Autodesk Inventor part; units mm, degrees
ref_plane "YZ Plane" through (0, 0, 0) normal (1, 0, 0) x (0, 1, 0)
ref_plane "XZ Plane" through (0, 0, 0) normal (0, 1, 0) x (-1, 0, 0)
ref_plane "XY Plane" through (0, 0, 0) normal (0, 0, 1) x (1, 0, 0)
sketch "Sketch1" plane through (0, 0, 0) normal (0, 1, 0) x (-1, 0, 0)
  line L0 (0, 0) -> (55, 0)
  line L1 (55, 0) -> (55, -63)
  line L2 (55, -63) -> (0, -63)
  line L3 (0, -63) -> (0, 0)
  dimension "d0" = 55
  dimension "d1" = 63
extrude "Extrusion1" add sketch "Sketch1" along normal blind 3
sketch "Sketch2" plane through (0, 0, 0) normal (0, -1, 0) x (1, 0, 0)
  line L0 (0, 0) -> (-10, 0)
  line L1 (-10, 0) -> (-10, -3)
  line L2 (-10, -3) -> (0, -3)
  line L3 (0, -3) -> (0, 0)
  line L4 (-55, -63) -> (-55, 0)
  line L5 (-55, 0) -> (-45, 0)
  line L6 (-45, 0) -> (-45, -3)
  line L7 (-45, -3) -> (-55, -3)
  line L8 (-55, -3) -> (-55, 0)
  line L9 (-55, -63) -> (-45, -63)
  line L10 (-45, -63) -> (-45, -60)
  line L11 (-45, -60) -> (-55, -60)
  line L12 (-55, -60) -> (-55, -63)
  line L13 (0, -63) -> (-10, -63)
  line L14 (-10, -63) -> (-10, -60)
  line L15 (-10, -60) -> (0, -60)
  line L16 (0, -60) -> (0, -63)
  dimension "d4" = 10
  dimension "d5" = 3
  dimension "d6" = 10
  dimension "d7" = 3
  dimension "d8" = 10
  dimension "d9" = 3
  dimension "d10" = 10
  dimension "d11" = 3
extrude "Extrusion2" add sketch "Sketch2" along normal blind 7
sketch "Sketch3" plane through (-55, 3, 0) normal (0, 0, 1) x (1, 0, 0)
  line L0 (10, -10) -> (0, -10)
  line L1 (0, -10) -> (5, -10)
  line L2 (5, -10) -> (5, -6)
  line L3 (5, -6) -> (0, -6)
  line L4 (0, -6) -> (0, -10)
  line L5 (45, -3) -> (45, -10)
  line L6 (45, -10) -> (50, -10)
  line L7 (50, -10) -> (50, -6)
  line L8 (50, -6) -> (45, -6)
  line L9 (45, -6) -> (45, -10)
  circle A0 centre (5, -6) radius 2
  circle A1 centre (50, -6) radius 2
  point P0 (55, -3)
  dimension "d14" = 5
  dimension "d15" = 4
  dimension "d16" = 5
  dimension "d17" = 4
  dimension "d18" = 4
  dimension "d19" = 4
extrude "Extrusion3" cut sketch "Sketch3" against normal up to surface (63 mm away) contours A0 L3 L2 | L2 L3 A0 | A1 L7 L8 | L8 L7 A1
fillet "Fillet1" radius 4 8 edges at (0, -7, -1.5) (-10, -7, -61.5) (0, -7, -61.5) (-45, -7, -61.5) (-55, -7, -61.5) (-45, -7, -1.5) (-55, -7, -1.5) (-10, -7, -1.5)
sketch "Sketch4" plane through (0, 3, 0) normal (0, 1, 0) x (1, 0, 0)
  line L0 (0, 0) -> (15, 0)
  line L1 (15, 0) -> (15, 63)
  line L2 (15, 63) -> (0, 63)
  line L3 (0, 63) -> (0, 0)
  dimension "d23" = 15
  dimension "d24" = 63
extrude "Extrusion4" add sketch "Sketch4" against normal blind 3
sketch "Sketch5" plane through (0, 3, 0) normal (0, 1, 0) x (1, 0, 0)
  line L0 (14.6866, 62.7723) -> (4.6866, 62.7723)
  line L1 (4.6866, 62.7723) -> (4.6866, 52.7723)
  line L2 (4.6866, 52.7723) -> (14.6866, 52.7723)
  line L3 (14.6866, 52.7723) -> (14.6866, 62.7723)
  line L4 (4.6866, 52.7723) -> (-25.6434, 52.7723)
  line L5 (-25.6434, 52.7723) -> (-25.6434, 37.0423)
  line L6 (-25.6434, 37.0423) -> (4.6866, 37.0423)
  line L7 (4.6866, 37.0423) -> (4.6866, 52.7723)
  circle A0 centre (-25.6434, 52.7723) radius 1
  circle A1 centre (4.6866, 37.0423) radius 1
  circle A2 centre (4.6866, 37.0423) radius 2
  circle A3 centre (-25.6434, 52.7723) radius 2
  point P0 (0, 0)
  dimension "d27" = 10
  dimension "d28" = 10
  dimension "d29" = 30.33
  dimension "d30" = 15.73
  dimension "d31" = 2
  dimension "d32" = 2
  dimension "d33" = 4
  dimension "d34" = 4
extrude "Extrusion5" cut sketch "Sketch5" against normal blind 3 contours A0 L5 L4 | L4 L5 A0 | A1 L6 L7 | L7 L6 A1
sketch "Sketch6" plane through (0, 3, 0) normal (0, 1, 0) x (1, 0, 0)
  line L0 (15, 63) -> (-55, 63)
  line L1 (-55, 63) -> (-55, 53)
  line L2 (-55, 53) -> (-35, 53)
  line L3 (-35, 53) -> (-35, 33)
  line L4 (-35, 33) -> (-55, 33)
  line L5 (-55, 33) -> (-55, 53)
  point P0 (0, 0)
  dimension "d37" = 10
  dimension "d38" = 20
  dimension "d39" = 20
extrude "Extrusion6" cut sketch "Sketch6" against normal blind 3
fillet "Fillet2" radius 4 4 edges at (-35, 1.5, -53) (-35, 1.5, -33) (-55, 1.5, -53) (-55, 1.5, -33)
fillet "Fillet3" radius 4 2 edges at (15, 1.5, 0) (15, 1.5, -63)
sketch "Sketch7" plane through (0, 3, 0) normal (0, 1, 0) x (1, 0, 0)
  line L0 (15, 0) -> (5, 0)
  line L1 (5, 0) -> (5, 10)
  line L2 (5, 10) -> (15, 10)
  line L3 (15, 10) -> (15, 0)
  line L4 (5, 10) -> (-50.626, 10)
  line L5 (-50.626, 10) -> (-50.626, 16.3068)
  line L6 (5, 16.3068) -> (5, 10)
  line L7 (5, 10) -> (-50.626, 10)
  line L8 (-50.626, 10) -> (-50.626, 29.05)
  line L9 (-50.626, 29.05) -> (5, 29.05)
  line L10 (5, 29.05) -> (5, 10)
  circle A0 centre (-50.626, 10) radius 1
  circle A1 centre (-50.626, 29.05) radius 1
  circle A2 centre (5, 29.05) radius 1
  circle A3 centre (5, 10) radius 1
  point P0 (0, 0)
  dimension "d44" = 10
  dimension "d45" = 10
  dimension "d48" = 55.626
  dimension "d49" = 19.05
  dimension "d50" = 2
  dimension "d51" = 2
  dimension "d52" = 2
  dimension "d53" = 2
extrude "Extrusion7" cut sketch "Sketch7" against normal blind 3 contours A3 L4 L1 | L1 L2 A3 | L2 L6 A3 | L4 A3 L6 | A0 L5 L4 | L4 L5 A0 | A2 L9 L10 | L10 L9 A2 | A1 L9 L8 | L8 L9 A1
sketch "Sketch8" plane through (0, 3, 0) normal (0, 1, 0) x (1, 0, 0)
  circle A0 centre (-25.6434, 52.7723) radius 1
  line L0 (-25.6434, 52.7723) -> (-21.6434, 52.7723)
  circle A1 centre (4.6866, 37.0423) radius 1
  line L1 (4.6866, 37.0423) -> (0.6866, 37.0423)
  line L2 (-21.6434, 52.7723) -> (0.6866, 52.7723)
  line L3 (0.6866, 52.7723) -> (0.6866, 37.0423)
  line L4 (0.6866, 37.0423) -> (-21.6434, 37.0423)
  line L5 (-21.6434, 37.0423) -> (-21.6434, 52.7723)
  point P0 (0, 0)
  dimension "d56" = 4
  dimension "d57" = 4
extrude "Extrusion8" cut sketch "Sketch8" against normal blind 10 contours L2 L3 L4 L5
sketch "Sketch9" plane through (0, 3, 0) normal (0, 1, 0) x (1, 0, 0)
  line L0 (-28.7673, 5.8913) -> (-14.8119, 5.8913)
  line L1 (-14.8119, 5.8913) -> (-14.8119, -0.376)
  line L2 (-14.8119, -0.376) -> (-28.7673, -0.376)
  line L3 (-28.7673, -0.376) -> (-28.7673, 5.8913)
  point P0 (0, 0)
extrude "Extrusion9" cut sketch "Sketch9" against normal blind 10
fillet "Fillet4" radius 2 2 edges at (-28.7673, 1.5, 0) (-14.8119, 1.5, 0)
sketch "Sketch11" plane through (0, 3, 0) normal (0, 1, 0) x (1, 0, 0)
  line L0 (17.0243, 33.2031) -> (8.6813, 33.2031)
  line L1 (8.6813, 33.2031) -> (8.6813, 57.6685)
  line L2 (8.6813, 57.6685) -> (17.0243, 57.6685)
  line L3 (17.0243, 57.6685) -> (17.0243, 33.2031)
  point P0 (0, 0)
extrude "Extrusion11" cut sketch "Sketch11" against normal blind 10
fillet "Fillet5" radius 2 2 edges at (15, 1.5, -57.6685) (15, 1.5, -33.2031)
properties part number "servo_driver_support"
Could you check a few things on this model? Use its own coordinates, in mm. A direction names the side the tool comes from. Give positions to 0.01 mm unless a question says otherwise; leave off trailing zeros. Order: outer loops, then holes, each group sorted by start corner. A loop starts at its lowest first (then second) coordinate and runs counter-clockwise, first axis right, second up.
Item 1: If we section it at C-C, the plane y = -6: Write out the boundary of the cut face in (x, z).
Item 2: If we section it at D-D, the plane z = -17.5: Write out the boundary of the cut face in (x, y).
Item 3: For faces 4 (the face through (-51, -5, -60)), 5 (the face through (-14.812, 2, -4)), 6 (the face through (-8.797, -5.859, -1.521)), 7 (the face through (5, 2, -11)), 8 (the face through (-4, -1, 0)), which set-ups out of +Z, -Z, +X, -X, +Y, -Y let a thin tool reach every point of the face, with its end or its side?
Item 4: I need wall thicknesses on line 1 (X direction, y = -3, z = -1.9); line 2 (X direction, y = 0.7, z = -29.05); line 3 (Z direction, x = -49, y = -5.75). Which ranges of each line are inside material? Lowest first, please.
Item 5: If we mould it in two halves opening along X, with no side actions, what happens to faces 1 (the face through (-6.6, -4.2, -1.5)), 2 (the face through (-35, 2, -43)), 3 (the face through (14.43, 1.52, -32.6))? For each: pulls with the +X half, pulls with the -X half, needs draft (parallel to the pull), parting line crosses it, or undercut.
Item 6: If we section it at B-B, the plane x = -25.5: Write out the boundary of the cut face in (y, z), plus the area to 3 significant figures.
Item 7: If we section it at A-A, the plane z = -10: Write out the boundary of the cut face in (x, y).
Item 8: I'm going to push flat-ended pins straight in: pin 1 (12 mm diameter, centred on x = -28.5, z = -56, fed in from -Y); pin 2 (1.5 mm diameter, centred on y = 2, z = -39.5, fed in from +X); pin 3 (3.5 mm diameter, centred on y = 1, z = -42, fed in from -X); pin 4 (1.6 mm diameter, centred on x = 4.69, z = -37.04, fed in from -Y). Where does each tip first touch, or does it pass through?
Values:
1. outline: (-53.65, -63) - (-46.35, -63) - (-46.35, -60) - (-53.65, -60) - close; (-53.65, -3) - (-46.35, -3) - (-46.35, 0) - (-53.65, 0) - close; (-8.65, -63) - (-1.35, -63) - (-1.35, -60) - (-8.65, -60) - close; (-8.65, -3) - (-1.35, -3) - (-1.35, 0) - (-8.65, 0) - close
2. outline: (-55, 0) - (15, 0) - (15, 3) - (-55, 3) - close
3. face 4: +X, -X, -Y
3. face 5: +Z, +Y, -Y
3. face 6: +Z, -Z, -Y
3. face 7: +Y, -Y
3. face 8: +Z, +X, -X, +Y, -Y
4. line 1: x = -55 to -52, -48 to -45, -10 to -7, -3 to 0
4. line 2: x = -55 to -51.63, -49.63 to 4, 6 to 15
4. line 3: z = -63 to -60, -3 to 0
5. face 1: undercut
5. face 2: pulls with the -X half
5. face 3: pulls with the +X half
6. outline: (0, -63) - (3, -63) - (3, -53.76) - (0, -53.76) - close; (0, -51.78) - (3, -51.78) - (3, -5.89) - (0, -5.89) - close
6. area: 165 mm2
7. outline: (-55, 0) - (-51.63, 0) - (-51.63, 3) - (-55, 3) - close; (-49.63, 0) - (4, 0) - (4, 3) - (-49.63, 3) - close; (6, 0) - (15, 0) - (15, 3) - (6, 3) - close
8. pin 1: stops at y = 0
8. pin 2: stops at x = 8.68
8. pin 3: stops at x = -35
8. pin 4: passes through
